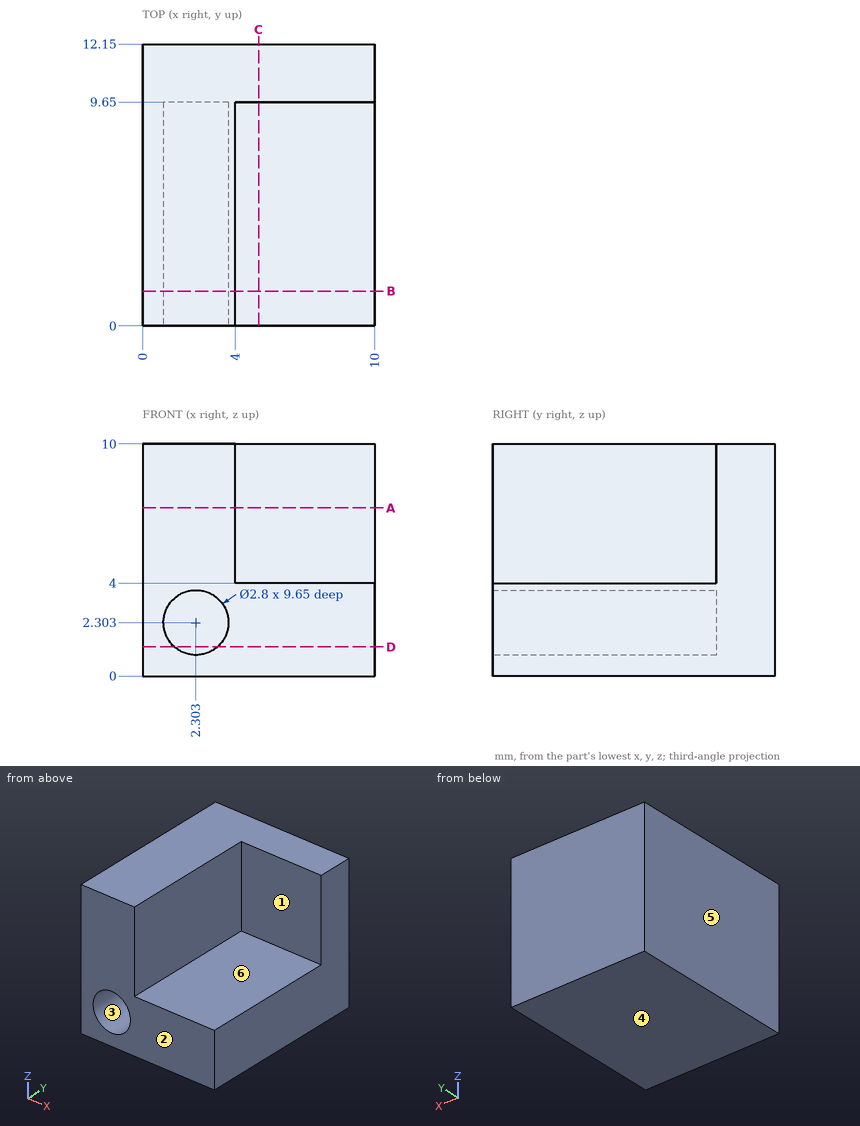
Answer from the drawing. Dimensions are ordinates in mm from the lowest x, y and z of the part. A direction names the side the tool comes from. Coordinates: 2 decimals unless noted, no trailing zeros. Write each loop counter-clockwise with the first axis right and the second up, starting at its lowest first coordinate (ties: lowest second). Pieces come first, ordered by that corner, then holes. Notation, with made-up numbers: M 21.5,18.25 L 54.5,18.25 A18 cw 54.5,34.25 Z; hole C 73.25,63 d1. An arc over 180 degrees is marked long. Use a Markdown table: item, result.
Q1. Straight lines are drawn through the part: L1, parallel to X at y = 4.5, z = 2.25; L2, parallel to Y at x = 8.25, z = 6; L3, parallel to X at y = 7, z = 4.5. For each, find the intervals that lie inside material, in ascending order. Write a range as [from, to].
Answer block:
| item | result |
|---|---|
| L1 | x = [0, 0.9], [3.7, 10] |
| L2 | y = [9.65, 12.15] |
| L3 | x = [0, 4] |
Q2. Determine the mould class of the marked faces 3, 4, 5 and 6 for opening direction Z: released by +Z, released by -Z, zero draft, split by the parting line, or undercut.
Answer block:
| item | result |
|---|---|
| face 3 | undercut |
| face 4 | released by -Z |
| face 5 | zero draft |
| face 6 | released by +Z |
Q3. The part is cut by section C-C, the plane x = 5. Write down the section's boundary in (y, z), then the cut area to 3 significant figures.
Answer block:
| item | result |
|---|---|
| outline | M 0,0 L 12.15,0 L 12.15,10 L 9.65,10 L 9.65,4 L 0,4 Z |
| area | 63.6 mm2 |
Q4. The part is cut by section A-A, the plane z = 7.25. Write down the section's boundary in (x, y), then the cut area to 3 significant figures.
Answer block:
| item | result |
|---|---|
| outline | M 0,0 L 4,0 L 4,9.65 L 10,9.65 L 10,12.15 L 0,12.15 Z |
| area | 63.6 mm2 |
Q5. The part is cut by section D-D, the plane z = 1.25. Write down the section's boundary in (x, y).
Answer block:
| item | result |
|---|---|
| outline | M 0,0 L 1.38,0 L 1.38,9.65 L 3.23,9.65 L 3.23,0 L 10,0 L 10,12.15 L 0,12.15 Z |
Q6. This flat-tipped pin is pushed along its axis until it touches: pin 1 Ø1.7 at (x, z) = (2.3, 2.3) entering from -Y. Where does it stop, or does it pass through?
Answer block:
| item | result |
|---|---|
| pin 1 | stops at y = 9.65 |
Q7. Which of the six approach directions +Z, -Z, +X, -X, +Y, -Y give full straight-line access (tool end or side, diameter ignored) to the marked faces 1 and 2?
Answer block:
| item | result |
|---|---|
| face 1 | +Z, +X, -Y |
| face 2 | +Z, -Z, +X, -X, -Y |
Q8. The part is cut by section B-B, the plane y = 1.5. Write down the section's boundary in (x, z), then the cut area to 3 significant figures.
Answer block:
| item | result |
|---|---|
| outline | M 0,0 L 10,0 L 10,4 L 4,4 L 4,10 L 0,10 Z; hole C 2.3,2.3 d2.8 |
| area | 57.8 mm2 |
